Geometry check sheet. Reference: the model listing, model coordinates, mm. A direction names the side the tool comes from. Round coordinates to 2 decimals unless told otherwise and drop trailing zeros. Write each loop counter-clockwise with the first axis right and the second up, starting at its lowest first coordinate (ties: lowest second). Pieces come first, ordered by that corner, then holes.
Item 1: Draft check along Y on faces 1 (the face through (2, 33.5, 10)), 2 (the face through (-14.79, 23.505, 10.22)), 3 (the face through (25.5, 24, 10)). Enter one of: pulls with the +Y half, pulls with the -Y half, needs draft (parallel to the pull), parting line crosses it, or undercut.
Item 2: Access from +Z, -Z, +X, -X, +Y, -Y to the whole of each face (thin tool, end or side, straight path). Record for faces 4 (the face through (4, 14, 5)), 5 (the face through (22, 28.5, 10)), 6 (the face through (30.43, 25.46, 9.86)), 7 (the face through (15, 4, 10)).
Item 3: Cross-section at D-D (x = -19.5). Enter the section's corners in (y, z).
Item 4: Cross-section at B-B (z = 17.25). Enter the section's corners in (x, y), then the cut area to 3 significant figures.
Item 5: Cross-section at C-C (y = 14.25). Enter the section's corners in (x, z).
Item 6: Depth check by flat-ended pin: P1, Ø10, axis at x = 17, z = 10, coming from the -Y side; P2, Ø2.5, axis at y = 12.5, z = 10, coming from the +X side; P3, Ø6, axis at x = -20.5, z = 4, coming from the -Y side; P4, Ø3, axis at x = 6, y = 16.5, coming from the +Z side. Enter the tip coordinate at first touch or a pass-through.
Item 7: Scan lines: probe 1 along Y at (x, z) = (17.5, 19.25); probe 2 along X at (y, z) = (20.5, 5.75); probe 3 along X at (y, z) = (29.5, 5.75). Record each from-to range of solid material in increasing order.
Item 8: Cross-section at A-A (x = 16.5). Enter the section's corners in (y, z), then the cut area to 3 significant figures.
from build123d import *

# Parameters (mm, degrees)
PAD_DEPTH    = 20
PAD003_DEPTH = 20
SKETCH001_R  = 5
PAD004_DEPTH = 30
SKETCH003_R  = 4
PAD005_DEPTH = 10


with BuildPart() as part:
    # Sketch → Pad (new body)
    with BuildSketch(Plane.XY):
        Polygon((0, 0), (35.5, 0), (25.5, 6), (25.5, 4), (4, 4), (4, 24.5), (25.5, 24.5), (25.5, 22.5), (35.5, 28.5), (0, 28.5), align=None)
    extrude(amount=PAD_DEPTH)

    # Sketch002 → Pad003 (join)
    with BuildSketch(Plane.XY):
        with BuildLine():
            Line((0, 33.5), (0, 28.5))
            Line((0, 28.5), (4, 28.5))
            Line((4, 28.5), (9.000029, 28.5))
            ThreePointArc((4, 33.5), (5.464476, 29.964456), (9.000029, 28.5))
            Line((4, 33.5), (0, 33.5))
        make_face()
    extrude(amount=PAD003_DEPTH)

    # Sketch001 → Pad004 (join)
    with BuildSketch(Plane.YZ):
        with Locations((28.5, 10)):
            Circle(SKETCH001_R)
    extrude(amount=-PAD004_DEPTH)

    # Sketch003 → Pad005 (join)
    with BuildSketch(Plane.YZ):
        with Locations((14.25, 10)):
            Circle(SKETCH003_R)
    extrude(amount=PAD005_DEPTH)


solid = part.part
Resolved:
1. face 1: pulls with the +Y half
1. face 2: parting line crosses it
1. face 3: undercut
2. face 4: none
2. face 5: +Z, -Z, +X, +Y
2. face 6: +Z, -Z, +X
2. face 7: +Z, -Z
3. outline: circle Ø10 at (28.5, 10)
4. outline: (0, 0) - (35.5, 0) - (25.5, 6) - (25.5, 4) - (4, 4) - (4, 24.5) - (25.5, 24.5) - (25.5, 22.5) - (35.5, 28.5) - (9, 28.5) arc R5 cw to (4, 33.5) - (0, 33.5) - close
4. area: 371 mm2
5. outline: (0, 0) - (4, 0) - (4, 6) - (10, 6) - (10, 14) - (4, 14) - (4, 20) - (0, 20) - close
6. P1: stops at y = 0
6. P2: stops at x = 10
6. P3: stops at y = 24.5
6. P4: stops at z = 13.93
7. probe 1: y = 0 to 4, 24.5 to 28.5
7. probe 2: x = 0 to 4
7. probe 3: x = -30 to 6
8. outline: (0, 0) - (4, 0) - (4, 20) - (0, 20) - close; (24.5, 0) - (28.5, 0) - (28.5, 20) - (24.5, 20) - close
8. area: 160 mm2
